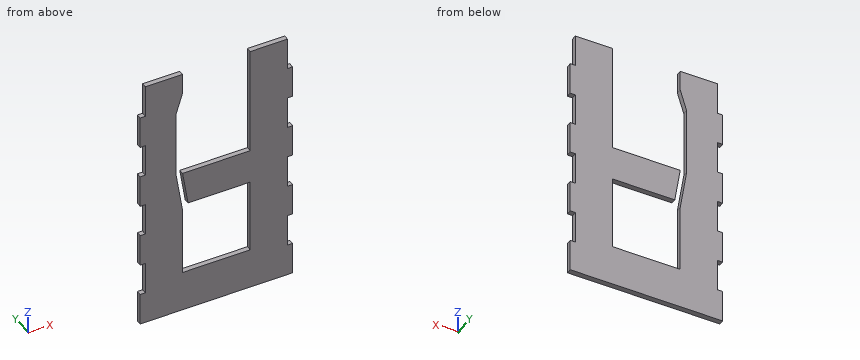
```python
from build123d import *

# Parameters (mm, degrees)
BOSS_EXTRUDE1_DEPTH = 3.175
SKETCH3_W           = 15
SKETCH3_H           = 20
SKETCH3_R           = 3.5
BOSS_EXTRUDE3_DEPTH = 3.175
SKETCH4_W           = 23.175
SKETCH4_H           = 6.096
BOSS_EXTRUDE4_DEPTH = 3.175
SKETCH5_W           = 11.825
SKETCH5_H           = 166.096
CUT_EXTRUDE1_DEPTH  = 191.502764088
SKETCH6_W           = 88.35
SKETCH6_H           = 6.096
CUT_EXTRUDE2_DEPTH  = 185.355380312


with BuildPart() as part:
    # Sketch1 → Boss-Extrude1 (new body)
    with BuildSketch(Plane(origin=(0, 0, 0), x_dir=(1, 0, 0), z_dir=(0, 1, 0))):
        Polygon((0, 160), (0, 0), (23.175, 0), (23.175, 12.666666667), (19.175, 25.333333333), (19.175, 67.333333333), (23.175, 92.666666667), (23.175, 134.666666667), (65.175, 134.666666667), (65.175, 92.666666667), (65.175, 88.666666667), (26.543421053, 88.666666667), (23.175, 67.333333333), (65.175, 67.333333333), (65.175, 25.333333333), (65.175, 0), (88.35, 0), (88.35, 160), align=None)
    extrude(amount=BOSS_EXTRUDE1_DEPTH)

    # Sketch3 → Boss-Extrude3 (add)
    # profile 1 of 8: a face of its own
    with BuildSketch(Plane(origin=(0, 3.175, 0), x_dir=(1, 0, 0), z_dir=(0, 1, 0))):
        with Locations((-7.5, 150)):
            Rectangle(SKETCH3_W, SKETCH3_H)
        with Locations(Location((-7.5, 150, 0), (0, 0, 270))):
            Circle(SKETCH3_R, mode=Mode.SUBTRACT)
    # profile 2 of 8: a face of its own
    with BuildSketch(Plane(origin=(0, 3.175, 0), x_dir=(1, 0, 0), z_dir=(0, 1, 0))):
        with Locations((-7.5, 110)):
            Rectangle(SKETCH3_W, SKETCH3_H)
        with Locations(Location((-7.5, 110, 0), (0, 0, 270))):
            Circle(SKETCH3_R, mode=Mode.SUBTRACT)
    # profile 3 of 8: a face of its own
    with BuildSketch(Plane(origin=(0, 3.175, 0), x_dir=(1, 0, 0), z_dir=(0, 1, 0))):
        with Locations((-7.5, 70)):
            Rectangle(SKETCH3_W, SKETCH3_H)
        with Locations(Location((-7.5, 70, 0), (0, 0, 270))):
            Circle(SKETCH3_R, mode=Mode.SUBTRACT)
    # profile 4 of 8: a face of its own
    with BuildSketch(Plane(origin=(0, 3.175, 0), x_dir=(1, 0, 0), z_dir=(0, 1, 0))):
        with Locations((-7.5, 30)):
            Rectangle(SKETCH3_W, SKETCH3_H)
        with Locations(Location((-7.5, 30, 0), (0, 0, 270))):
            Circle(SKETCH3_R, mode=Mode.SUBTRACT)
    # profile 5 of 8: a face of its own
    with BuildSketch(Plane(origin=(0, 3.175, 0), x_dir=(1, 0, 0), z_dir=(0, 1, 0))):
        with Locations((95.85, 30)):
            Rectangle(SKETCH3_W, SKETCH3_H)
        with Locations(Location((95.85, 30, 0), (0, 0, 270))):
            Circle(SKETCH3_R, mode=Mode.SUBTRACT)
    # profile 6 of 8: a face of its own
    with BuildSketch(Plane(origin=(0, 3.175, 0), x_dir=(1, 0, 0), z_dir=(0, 1, 0))):
        with Locations((95.85, 70)):
            Rectangle(SKETCH3_W, SKETCH3_H)
        with Locations(Location((95.85, 70, 0), (0, 0, 270))):
            Circle(SKETCH3_R, mode=Mode.SUBTRACT)
    # profile 7 of 8: a face of its own
    with BuildSketch(Plane(origin=(0, 3.175, 0), x_dir=(1, 0, 0), z_dir=(0, 1, 0))):
        with Locations((95.85, 110)):
            Rectangle(SKETCH3_W, SKETCH3_H)
        with Locations(Location((95.85, 110, 0), (0, 0, 270))):
            Circle(SKETCH3_R, mode=Mode.SUBTRACT)
    # profile 8 of 8: a face of its own
    with BuildSketch(Plane(origin=(0, 3.175, 0), x_dir=(1, 0, 0), z_dir=(0, 1, 0))):
        with Locations((95.85, 150)):
            Rectangle(SKETCH3_W, SKETCH3_H)
        with Locations(Location((95.85, 150, 0), (0, 0, 270))):
            Circle(SKETCH3_R, mode=Mode.SUBTRACT)
    extrude(amount=-BOSS_EXTRUDE3_DEPTH)

    # Sketch4 → Boss-Extrude4 (add)
    with BuildSketch(Plane(origin=(0, 3.175, 0), x_dir=(1, 0, 0), z_dir=(0, 1, 0))):
        with Locations((11.5875, -3.048)):
            Rectangle(SKETCH4_W, SKETCH4_H)
        with Locations((76.7625, -3.048)):
            Rectangle(SKETCH4_W, SKETCH4_H)
    extrude(amount=-BOSS_EXTRUDE4_DEPTH)

    # Sketch5 → Cut-Extrude1 (cut, through all)
    with BuildSketch(Plane(origin=(0, 3.175, 0), x_dir=(1, 0, 0), z_dir=(0, 1, 0))):
        with Locations((-9.0875, 76.952)):
            Rectangle(SKETCH5_W, SKETCH5_H)
        with Locations((97.4375, 76.952)):
            Rectangle(SKETCH5_W, SKETCH5_H)
    extrude(amount=-CUT_EXTRUDE1_DEPTH, mode=Mode.SUBTRACT)

    # Sketch6 → Cut-Extrude2 (cut, through all)
    with BuildSketch(Plane(origin=(0, 3.175, 0), x_dir=(1, 0, 0), z_dir=(0, 1, 0))):
        with Locations((44.175, -3.048)):
            Rectangle(SKETCH6_W, SKETCH6_H)
    extrude(amount=-CUT_EXTRUDE2_DEPTH, mode=Mode.SUBTRACT)


solid = part.part
```
Here's how the part is built. I have some questions about the finished solid (model axes, mm). Coordinates: 2 decimals unless noted, no trailing zeros. Order: outer loops, then holes, each group sorted by start corner. A loop starts at its lowest first (then second) coordinate and runs counter-clockwise, first axis right, second up.
Item 1: If we section it at A-A, the plane x = 59: List the corners of the cut face in (y, z) for me (3 decimals).
Response values:
outline: (0, -160) - (3.175, -160) - (3.175, -134.667) - (0, -134.667) - close; (0, -88.667) - (3.175, -88.667) - (3.175, -67.333) - (0, -67.333) - close
Item 2: I'm going to push flat-ended pins straight in: pin 1 Ø1.6 at (x, y) = (-2.5, 2) entering from +Z; pin 2 Ø1.6 at (x, y) = (46, 1) entering from +Z; pin 3 Ø1.6 at (y, z) = (1, -8.5) entering from +X. Where does each tip first touch, or does it pass through?
Response values:
pin 1: stops at z = -20
pin 2: stops at z = -67.33
pin 3: stops at x = 88.35
Item 3: If we section it at B-B, the plane z = -36: List the corners of the cut face in (x, y) for me (3 decimals), then the cut area to 3 significant figures.
Response values:
outline: (-3.175, 0) - (19.175, 0) - (19.175, 3.175) - (-3.175, 3.175) - close; (65.175, 0) - (91.525, 0) - (91.525, 3.175) - (65.175, 3.175) - close
area: 155 mm2
Item 4: I need wall thicknesses on probe 1 along Z at (x, y) = (59, 0.3); probe 2 along X at (y, z) = (2.5, -66) (3 decimals); probe 3 along X at (y, z) = (0.85, -97) (3 decimals). Which ranges of each line are inside material? Lowest first, please.
Response values:
probe 1: z = -160 to -134.67, -88.67 to -67.33
probe 2: x = -3.175 to 19.175, 65.175 to 91.525
probe 3: x = 0 to 23.175, 65.175 to 88.35
